Design review of the part shown in the three views and the two pictorial views. Dimensions are in mm from the part's minimum x, y and z. Give positions to 0.01 mm unless a question says otherwise; leave off trailing zeros. Loops run counter-clockwise (first coordinate to the right, second up) from the corner with the lowest first, then second, coordinate; pieces in that order, holes last. Notation, with made-up numbers: (67.25, 5.5) - (101.25, 5.5) arc R20 cw to (101.25, 34.5) - close; hole circle Ø10 at (20, -20). An arc over 180 degrees is marked (long way). Put each result on its own line as item: value. Start each with the question number.
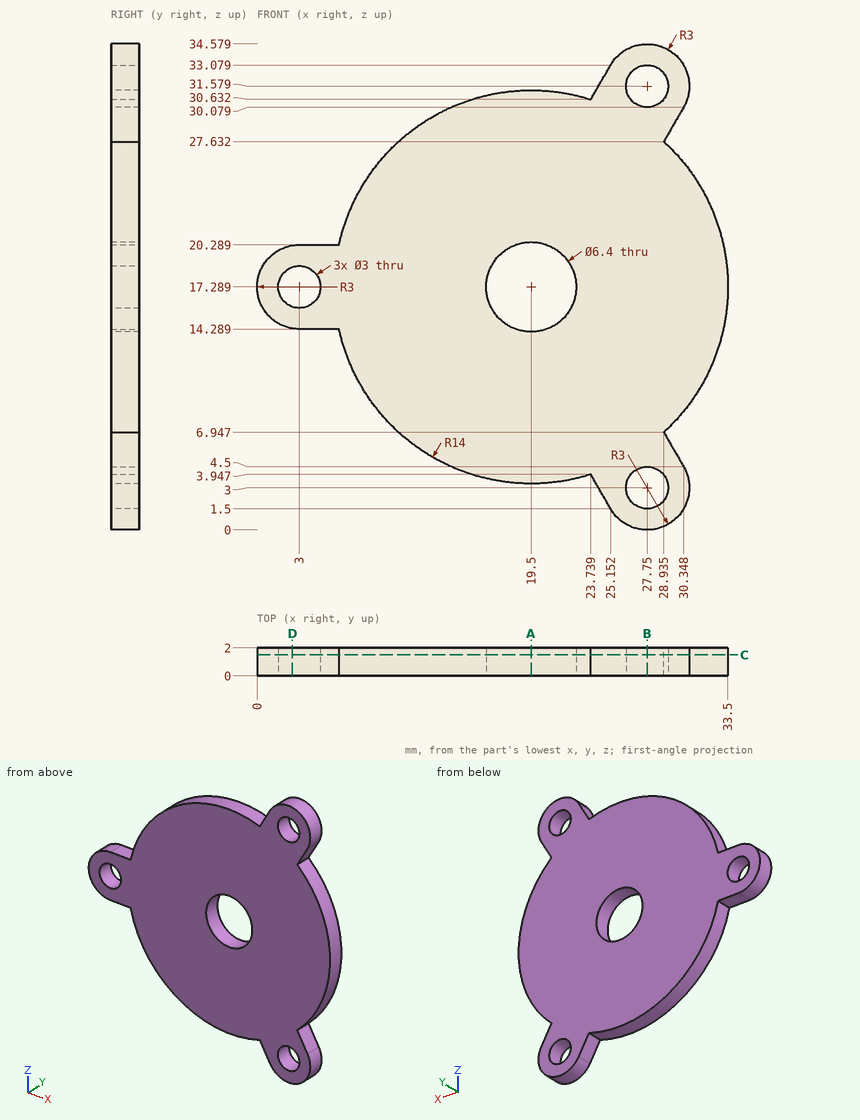
1) Take a section at D-D on x = 2.5. State the section outline as (y, z) points (1 decimal).
2) Take a section at B-B on x = 27.75. State the section outline as (y, z) points.
3) Insertion check: P1, Ø4, axis at x = 28, z = 19.5, coming from the -Y side; P2, Ø0.6, axis at x = 5, y = 1, coming from the -Z side; P3, Ø1.5, axis at x = 18.5, z = 17, coming from the -Y side; P4, Ø1, axis at y = 1.5, z = 25.5, coming from the -X side (1 decimal). Each pin has a flat end and moves straight along its axis. Give the tip position at first contact, or say it passes through.
4) Take a section at A-A on x = 19.5. State the section outline as (y, z) points.
5) Take a section at C-C on y = 1.5. State how many separate pieces and enclosed holes the cut face has, and give its area (3 significant figures).
6) Wall thickness on probe 1 along Z at (x, y) = (27, 0.85) (1 decimal); probe 2 along Z at (x, y) = (27.5, 1.1); probe 3 along Z at (x, y) = (4, 1) (1 decimal): over which ranges is each line inside the solid? List them lowest first.
Answers follow:
1. outline: (0, 14.3) - (2, 14.3) - (2, 15.9) - (0, 15.9) - close; (0, 18.7) - (2, 18.7) - (2, 20.2) - (0, 20.2) - close
2. outline: (0, 0) - (2, 0) - (2, 1.5) - (0, 1.5) - close; (0, 4.5) - (2, 4.5) - (2, 30.08) - (0, 30.08) - close; (0, 33.08) - (2, 33.08) - (2, 34.58) - (0, 34.58) - close
3. P1: y = 0
3. P2: z = 14.29
3. P3: through
3. P4: x = 7.8
4. outline: (0, 3.29) - (2, 3.29) - (2, 14.09) - (0, 14.09) - close; (0, 20.49) - (2, 20.49) - (2, 31.29) - (0, 31.29) - close
5. separate pieces: 1
5. enclosed holes: 4
5. area: 652 mm2
6. probe 1: 0.1 to 1.7, 4.3 to 30.3, 32.9 to 34.5
6. probe 2: 0.01 to 1.52, 4.48 to 30.1, 33.06 to 34.57
6. probe 3: 14.3 to 16.2, 18.4 to 20.3
